Input: part model. Units: mm. Frame: model coordinates. Face numbers are marked on the shaded views. A direction names the side the tool comes from. Give positions to 0.01 mm unless a question says otherwise; leave off trailing zeros. Loops run counter-clockwise (first coordinate to the right, second up) from the corner with the lowest first, then second, coordinate; pieces in that order, holes last. Notation, with made-up numbers: (50, 69) -> (59, 69) arc R22 ccw to (59, 79) -> close; hole circle Ø10 at (-2.5, 73.25). An arc over 180 degrees is marked (long way). Answer as a JSON object with one key per item and string values. Group by question number.
```python
from build123d import *

# Parameters (mm, degrees)
SKETCH_1_W             = 96
SKETCH_1_H             = 31
SKETCH_1_W_2           = 90
SKETCH_1_H_2           = 25
EXTRUDE_1_DEPTH        = 20
SKETCH_2_W             = 42.974010058
SKETCH_2_H             = 8.5
CUT_EXTRUDE_1_DEPTH    = 15
SKETCH_3_W             = 3
SKETCH_3_H             = 65.210399997
CUT_EXTRUDE_1_2_DEPTH  = 19
EXTRUDE_1_2_DEPTH      = 30
FILLET_1_R             = 1
FILLET_1_OF_MIRROR_2_R = 1


with BuildPart() as part:
    # 草图1 → Extrude 1 (new body)
    with BuildSketch(Plane.XY):
        Rectangle(SKETCH_1_W, SKETCH_1_H)
        Rectangle(SKETCH_1_W_2, SKETCH_1_H_2, mode=Mode.SUBTRACT)
    extrude(amount=EXTRUDE_1_DEPTH)

    # 草图2 → Cut-Extrude 1 (cut)
    with BuildSketch(Plane.XY.offset(20)):
        with Locations((45, 0)):
            Rectangle(SKETCH_2_W, SKETCH_2_H)
    extrude(amount=-CUT_EXTRUDE_1_DEPTH, mode=Mode.SUBTRACT)

    # 草图3 → Cut-Extrude 1 2 (cut)
    with BuildSketch(Plane.XY.offset(20)):
        with Locations((-14.5, 3.518261773)):
            Rectangle(SKETCH_3_W, SKETCH_3_H)
        with Locations((18.5, 3.518261773)):
            Rectangle(SKETCH_3_W, SKETCH_3_H)
    extrude(amount=-CUT_EXTRUDE_1_2_DEPTH, mode=Mode.SUBTRACT)

    # 草图4 → Extrude 1 2 (add)
    with BuildSketch(Plane.ZY.offset(13)):
        Polygon((20, 15.5), (22.5, 15.5), (22.5, 10.5), (20, 12.5), align=None)
    extrude_1_2 = extrude(amount=-EXTRUDE_1_2_DEPTH)

    # 圆角1
    fillet_1_edges = [part.edges().sort_by_distance(p)[0] for p in [
        (2, 10.5, 22.5),
    ]]
    fillet(fillet_1_edges, radius=FILLET_1_R)

    # 镜向2: Extrude 1 2 across plane
    add(extrude_1_2.mirror(Plane.ZX))

    # 圆角1 of 镜向2
    fillet_1_of_mirror_2_edges = [part.edges().sort_by_distance(p)[0] for p in [
        (2, -10.5, 22.5),
    ]]
    fillet(fillet_1_of_mirror_2_edges, radius=FILLET_1_OF_MIRROR_2_R)


solid = part.part
```
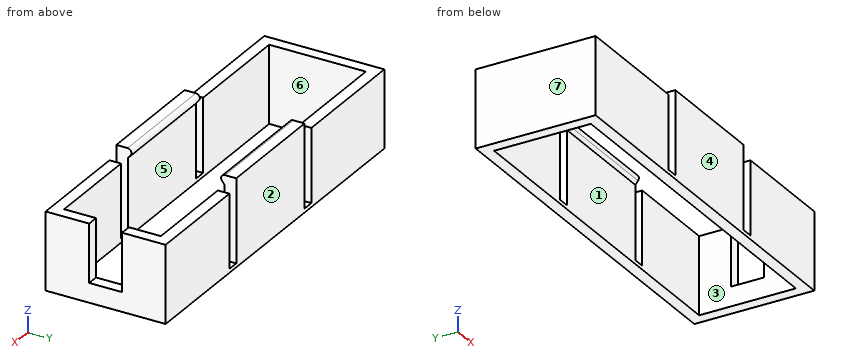
Q1. Set-up query: the marked faces 1, 2 and 3. Return all of +Z, -Z, +X, -X, +Y, -Y with unobstructed straight access to the full face (end or side cutting, diameter ignored); none if empty.
Q2. Section C-C on z = 11. Return the cut outline in (x, y), then the cut area to 4 significant figures.
Q3. Section B-B on y = 6. Return the cut outline in (x, z).
Q4. Section D-D on x = -6. Return the cut outline in (y, z).
Q5. Pin query (flat end, axial travel): pin 1 Ø12.5 at (x, y) = (30.5, 12.5) entering from +Z; pin 2 Ø3.5 at (x, y) = (46.5, -1) entering from +Z; pin 3 Ø1.5 at (x, y) = (-14.5, 13.5) entering from +Z. Return the tip coordinate at first contact, or that it passes through.
Q6. Ray query, probe 1 along Y at (x, z) = (1, 13.5); probe 2 along X at (y, z) = (-5, 3.5); probe 3 along X at (y, z) = (13.5, 7.5). Return the intervals inside material, ascending.
Q7. Section A-A on x = -20. Return the cut outline in (y, z).
Q8. Pull-direction query (X, two-part tool) for the marked faces 4, 5, 6 and 7; classes: +X half, -X half, draft (parallel to the pull), parting line (faces both ways), or undercut.
Numbers:
{
 "1": {"face 1": "-Z", "face 2": "+Z, -Z, +X, -X, +Y", "face 3": "+Z, -Z"},
 "2": {"outline": "(-48, -15.5) -> (-16, -15.5) -> (-16, -12.5) -> (-45, -12.5) -> (-45, 12.5) -> (-16, 12.5) -> (-16, 15.5) -> (-48, 15.5) -> close; (-13, -15.5) -> (17, -15.5) -> (17, -12.5) -> (-13, -12.5) -> close; (-13, 12.5) -> (17, 12.5) -> (17, 15.5) -> (-13, 15.5) -> close; (20, -15.5) -> (48, -15.5) -> (48, -4.25) -> (45, -4.25) -> (45, -12.5) -> (20, -12.5) -> close; (20, 12.5) -> (45, 12.5) -> (45, 4.25) -> (48, 4.25) -> (48, 15.5) -> (20, 15.5) -> close", "area": "664.5 mm²"},
 "3": {"outline": "(-48, 0) -> (-45, 0) -> (-45, 20) -> (-48, 20) -> close; (45, 0) -> (48, 0) -> (48, 20) -> (45, 20) -> close"},
 "4": {"outline": "(-15.5, 0) -> (-12.5, 0) -> (-12.5, 20) -> (-11.8, 20.88) arc R1 ccw to (-12.58, 22.5) -> (-15.5, 22.5) -> close; (11.8, 20.88) -> (12.5, 20) -> (12.5, 0) -> (15.5, 0) -> (15.5, 22.5) -> (12.58, 22.5) arc R1 ccw to start"},
 "5": {"pin 1": "stops at z = 20", "pin 2": "stops at z = 5", "pin 3": "stops at z = 1"},
 "6": {"probe 1": "y = -15.5 to -12.5, 12.5 to 15.5", "probe 2": "x = -48 to -45, 45 to 48", "probe 3": "x = -48 to -16, -13 to 17, 20 to 48"},
 "7": {"outline": "(-15.5, 0) -> (-12.5, 0) -> (-12.5, 20) -> (-15.5, 20) -> close; (12.5, 0) -> (15.5, 0) -> (15.5, 20) -> (12.5, 20) -> close"},
 "8": {"face 4": "draft", "face 5": "undercut", "face 6": "undercut", "face 7": "-X half"}
}
